Here's how the part is built. I have some questions about the finished solid (model axes, mm). A direction names the side the tool comes from. Coordinates: 2 decimals unless noted, no trailing zeros. Write each loop counter-clockwise with the first axis right and the second up, starting at its lowest first coordinate (ties: lowest second). Pieces come first, ordered by that corner, then holes. Notation, with made-up numbers: (76.5, 81) -> (82.5, 81) arc R19 ccw to (82.5, 106) -> close; hole circle Ø10 at (35.5, 10.25). An arc over 180 degrees is marked (long way). Use a Markdown table: item, result. Add a question column.
```python
from build123d import *

# Parameters (mm, degrees)
F1_DEPTH = 33
F2_ANGLE = 90
F3_T     = -4
F4_ANGLE = -90
F5_START = -4
F5_DEPTH = 25


with BuildPart() as f1:
    # F0 (on Front) → F1 (new body)
    with BuildSketch(Plane.XZ):
        Polygon((0, 40), (0, 0), (136.249770642, 0), align=None)
    extrude(amount=F1_DEPTH)


with BuildPart() as f1_1:
    # F2: moved
    add(f1.part.rotate(Axis((68.124885321, 0, 0), (-1, 0, 0)), F2_ANGLE))

    # F3 (hollow: no face is removed)
    offset(amount=F3_T, mode=Mode.SUBTRACT)


with BuildPart() as f1_2:
    # F4: moved
    add(f1_1.part.rotate(Axis((68.124885321, 0, 0), (-1, 0, 0)), F4_ANGLE))

    # F1_face (on face) → F5 (intersect)
    with BuildSketch(Plane(origin=(45.416590214, -33, 13.3333333333), x_dir=(1, 0, 0), z_dir=(0, -1, 0)).offset(F5_START)):
        Polygon((-45.416590214, 26.6666666667), (-45.416590214, -13.3333333333), (90.833180428, -13.3333333333), align=None)
    extrude(amount=-F5_DEPTH, mode=Mode.INTERSECT)


solid = f1_2.part
```
Q1. Will this pin go through, and if not, where does the flat tip stop? pin 1 (10 mm diameter, centred on x = 14, z = 23.5, fed in from +Y).
Q2. Thinking about a two-plate mould opening in Z: for faces 3 (the flat face through (4, -16, 20)), 4 (the flat face through (67, -17, 0)), 5 (the flat face through (69.08, -16.68, 19.72)), 6 (the flat face through (0, -17, 20)), which applies, released by +Z, released by -Z, zero draft, split by the parting line, or undercut?
Q3. Which directions (+Z, -Z, +X, -X, +Y, -Y) give clear straight access to the entire face, cutting with the end or side of a thin tool? Please do faces 1 (the flat face through (52.7, -29, 3.8)), 2 (the flat face through (55, -16, 4)).
Q4. Suppose I cut it at A-A, the plane y = -23.25. Write out the boundary of the cut face in (x, z), and give its area (3 significant figures).
Q5. Please list where these lines run through material, in increasing order: line 1 (Z direction, x = 85.5, y = -14.5); line 2 (Z direction, x = 35, y = -9); line 3 (Z direction, x = 122.5, y = -19.25).
Q6. Suppose I cut it at C-C, the plane x = 93.5. Write out the boundary of the cut face in (y, z).
Q7. Suppose I cut it at B-B, the plane z = 10. Write out the boundary of the cut face in (x, y), and give its area (3 significant figures).
Answer key:
| question | item | result |
|---|---|---|
| 1 | pin 1 | passes through |
| 2 | face 3 | undercut |
| 2 | face 4 | released by -Z |
| 2 | face 5 | released by +Z |
| 2 | face 6 | zero draft |
| 3 | face 1 | +Z, -Z, +X, -X, -Y |
| 3 | face 2 | +Y, -Y |
| 4 | outline | (0, 0) -> (136.25, 0) -> (0, 40) -> close; hole (4, 4) -> (108.42, 4) -> (4, 34.66) -> close |
| 4 | area | 1,120 mm^2 |
| 5 | line 1 | z = 0 to 4, 10.73 to 14.9 |
| 5 | line 2 | z = 0 to 4, 25.56 to 29.72 |
| 5 | line 3 | z = 0 to 4.04 |
| 6 | outline | (-29, 0) -> (-4, 0) -> (-4, 4) -> (-29, 4) -> close; (-29, 8.38) -> (-4, 8.38) -> (-4, 12.55) -> (-29, 12.55) -> close |
| 7 | outline | (0, -29) -> (4, -29) -> (4, -4) -> (0, -4) -> close; (87.99, -29) -> (102.19, -29) -> (102.19, -4) -> (87.99, -4) -> close |
| 7 | area | 455 mm^2 |
